from build123d import *

# Parameters (mm, degrees)
SKETCH1_W           = 147.32
SKETCH1_H           = 5.08
BOSS_EXTRUDE1_DEPTH = 172.72
SKETCH2_R           = 2.159
CUT_EXTRUDE1_DEPTH  = 6.08
SKETCH3_W           = 59.69
SKETCH3_H           = 96.52
BOSS_EXTRUDE2_DEPTH = 2.54
SKETCH4_W           = 2.54
SKETCH4_H           = 96.52
BOSS_EXTRUDE3_DEPTH = 25.4
SKETCH5_W           = 76.2
SKETCH5_H           = 22.86
BOSS_EXTRUDE4_DEPTH = 17.78
CUT_EXTRUDE2_DEPTH  = 150.86
SKETCH7_R           = 2
CUT_EXTRUDE3_DEPTH  = 28.94


with BuildPart() as part:
    # Sketch1 → Boss-Extrude1 (new body)
    with BuildSketch(Plane.XY):
        Rectangle(SKETCH1_W, SKETCH1_H)
    extrude(amount=BOSS_EXTRUDE1_DEPTH)

    # Sketch2 → Cut-Extrude1 (cut, through all)
    with BuildSketch(Plane(origin=(0, 2.54, 0), x_dir=(1, 0, 0), z_dir=(0, 1, 0))):
        with Locations((62.738, -12.7)):
            Circle(SKETCH2_R)
        with Locations((-62.865, -160.02)):
            Circle(SKETCH2_R)
        with Locations((62.865, -160.02)):
            Circle(SKETCH2_R)
        with Locations((-62.738, -12.7)):
            Circle(SKETCH2_R)
    extrude(amount=-CUT_EXTRUDE1_DEPTH, mode=Mode.SUBTRACT)

    # Sketch3 → Boss-Extrude2 (add)
    with BuildSketch(Plane(origin=(0, 2.54, 0), x_dir=(1, 0, 0), z_dir=(0, 1, 0))):
        with Locations((-18.415, -111.76)):
            Rectangle(SKETCH3_W, SKETCH3_H)
    extrude(amount=BOSS_EXTRUDE2_DEPTH)

    # Sketch4 → Boss-Extrude3 (add)
    with BuildSketch(Plane(origin=(0, 5.08, 0), x_dir=(1, 0, 0), z_dir=(0, 1, 0))):
        with Locations((-46.99, -111.76)):
            Rectangle(SKETCH4_W, SKETCH4_H)
    extrude(amount=BOSS_EXTRUDE3_DEPTH)

    # Sketch5 → Boss-Extrude4 (add)
    with BuildSketch(Plane.ZY.offset(48.26)):
        with Locations((111.76, 13.97)):
            Rectangle(SKETCH5_W, SKETCH5_H)
    extrude(amount=BOSS_EXTRUDE4_DEPTH)

    # Sketch6 → Cut-Extrude2 (cut, through all)
    with BuildSketch(Plane.XY.offset(149.86)):
        Polygon((-66.04, 2.54), (-48.26, 25.4), (-66.04, 25.4), align=None)
        Polygon((-61.213257367, 2.54), (-48.26, 19.194188043), (-48.26, 2.54), align=None)
    extrude(amount=-CUT_EXTRUDE2_DEPTH, mode=Mode.SUBTRACT)

    # Sketch7 → Cut-Extrude3 (cut, through all)
    with BuildSketch(Plane(origin=(-45.72, 0, 0), x_dir=(0, 0, -1), z_dir=(1, 0, 0))):
        with Locations((-155.26, 16.83)):
            Circle(SKETCH7_R)
        with Locations((-68.26, 16.83)):
            Circle(SKETCH7_R)
    extrude(amount=-CUT_EXTRUDE3_DEPTH, mode=Mode.SUBTRACT)


solid = part.part
Geometry: final body of the model. Coordinates: model frame, mm. A direction names the side the tool comes from. Give positions to 0.01 mm unless a question says otherwise; leave off trailing zeros. Write each loop counter-clockwise with the first axis right and the second up, starting at its lowest first coordinate (ties: lowest second). Pieces come first, ordered by that corner, then holes. Notation, with made-up numbers: M 17.5,10 L 48.5,10 A26 cw 48.5,29 Z; hole C -26.75,81 d9. An arc over 180 degrees is marked long. Answer in a Markdown table with one row per item. Add a question column.
(1) Section D-D on y = 12. Return loops of the section in (x, z), and give its area (3 significant figures).
(2) First-contact query: pin 1 (1.5 mm diameter, centred on x = 34.5, z = 127, fed in from +Y); pin 2 (5 mm diameter, centred on y = 16.83, z = 155.26, fed in from -X); pin 3 (19.5 mm diameter, centred on x = -55, y = 16, fed in from -Z); pin 4 (7 mm diameter, centred on x = -62.738, z = 12.7, fed in from -Y). Flat tips, straight axial feed; report the tip coordinate or a pass-through.
(3) Section A-A on z = 68.26. Return loops of the section in (x, y), and give its area (3 significant figures).
(4) Reachability of faces 4 (the flat face through (-27, 4, 160.02)), 5 (the cylindrical face through (64.86, 0.04, 160.85)), 6 (the flat face through (-56, 12, 149.86)), 7 (the flat face through (-18, 5.08, 111)) from +Z, -Z, +X, -X, +Y, -Y: full face, straight path, thin tool, end or side. Return the list, or none.
(5) Mould query, pull axis Y, two halves, no side actions, for faces 1 (the flat face through (-73.66, 0, 85)), 2 (the flat face through (-57.274, 13.81, 112.293)), 3 (the flat face through (-48.26, 16, 112)). Classes: +Y half, -Y half, draft (parallel to the pull), parting line (faces both ways), or undercut.
(6) Ray query, line 1 (X direction, y = -0.3, z = 12.7); line 2 (Y direction, x = -48, z = 154.5); line 3 (Y direction, x = 63.5, z = 92). Return the intervals inside material, ascending.
(7) Section C-C on z = 147.5. Return loops of the section in (x, y).
(8) Section B-B on z = 12.7. Return loops of the section in (x, y), and give its area (3 significant figures).
Result set:
| question | item | result |
|---|---|---|
| 1 | outline | M -58.68,73.66 L -53.86,73.66 L -53.86,149.86 L -58.68,149.86 Z; M -48.26,63.5 L -45.72,63.5 L -45.72,160.02 L -48.26,160.02 Z |
| 1 | area | 613 mm^2 |
| 2 | pin 1 | stops at y = 2.54 |
| 2 | pin 2 | stops at x = -48.26 |
| 2 | pin 3 | stops at z = 63.5 |
| 2 | pin 4 | stops at y = -2.54 |
| 3 | outline | M -73.66,-2.54 L 73.66,-2.54 L 73.66,2.54 L 11.43,2.54 L 11.43,5.08 L -45.72,5.08 L -45.72,14.83 L -48.26,14.83 L -48.26,2.54 L -73.66,2.54 Z; M -48.26,18.83 L -45.72,18.83 L -45.72,30.48 L -48.26,30.48 Z |
| 3 | area | 954 mm^2 |
| 4 | face 4 | +Z, +X, -X, +Y |
| 4 | face 5 | +Y, -Y |
| 4 | face 6 | +Z, -X, +Y |
| 4 | face 7 | +Z, -Z, +X, +Y |
| 5 | face 1 | draft |
| 5 | face 2 | +Y half |
| 5 | face 3 | undercut |
| 6 | line 1 | x = -73.66 to -64.9, -60.58 to 60.58, 64.9 to 73.66 |
| 6 | line 2 | y = -2.54 to 14.98, 18.68 to 30.48 |
| 6 | line 3 | y = -2.54 to 2.54 |
| 7 | outline | M -73.66,-2.54 L 73.66,-2.54 L 73.66,2.54 L 11.43,2.54 L 11.43,5.08 L -45.72,5.08 L -45.72,30.48 L -48.26,30.48 L -48.26,25.4 L -66.04,2.54 L -73.66,2.54 Z; hole M -61.21,2.54 L -48.26,2.54 L -48.26,19.19 Z |
| 8 | outline | M -73.66,-2.54 L -64.9,-2.54 L -64.9,2.54 L -73.66,2.54 Z; M -60.58,-2.54 L 60.58,-2.54 L 60.58,2.54 L -60.58,2.54 Z; M 64.9,-2.54 L 73.66,-2.54 L 73.66,2.54 L 64.9,2.54 Z |
| 8 | area | 705 mm^2 |
